Design review of the part built by this model. Coordinates are the model's own, in mm. Round coordinates to 2 decimals unless told otherwise and drop trailing zeros. Order: outer loops, then holes, each group sorted by start corner. A loop starts at its lowest first (then second) coordinate and runs counter-clockwise, first axis right, second up. Notation, with made-up numbers: M 37,5.25 L 41,5.25 A29 cw 41,33.25 Z; hole C 55,1.25 d9. An arc over 180 degrees is marked long. Write each question's results on one line, items separated by ' | '. Start each with the question number.
Item 1: Take a section at A-A, the plane x = 20.5. Write out the cut boundary in (y, z), plus the area to 3 significant figures.
Item 2: Take a section at B-B, the plane y = -41. Write out the cut boundary in (x, z) (3 decimals).
Item 3: Wall thickness on line 1 (X direction, y = 40, z = 2.5); line 2 (Y direction, x = 41.5, z = 4.5): over which ranges is each line inside the solid? List them lowest first. Write a range as [from, to].
Item 4: Clearance check with flat-ended pins moving along their axes: pin 1 (10 mm diameter, centred on x = -17, y = 2, fed in from -Z); pin 2 (3 mm diameter, centred on x = 41, y = 41, fed in from +Z). State where each tip first meets the part, or that it passes through.
```python
from build123d import *

# Parameters (mm, degrees)
F0_R     = 1.725
F0_W     = 3.5
F0_H     = 3.5
F1_DEPTH = 10


with BuildPart() as f1:
    # F0 (on Top) → F1 (new body)
    with BuildSketch(Plane.XY):
        Polygon((45, -45), (45, 0), (45, 45), (0, 45), (-45, 45), (-45, 0), (-45, -45), (0, -45), align=None)
        with Locations((-41, -41)):
            Circle(F0_R, mode=Mode.SUBTRACT)
        with Locations((-20, -20)):
            Rectangle(F0_W, F0_H, mode=Mode.SUBTRACT)
        with Locations((41, -41)):
            Circle(F0_R, mode=Mode.SUBTRACT)
        with Locations((20, -20)):
            Rectangle(F0_W, F0_H, mode=Mode.SUBTRACT)
        with Locations((-20, 20)):
            Rectangle(F0_W, F0_H, mode=Mode.SUBTRACT)
        with Locations((-41, 41)):
            Circle(F0_R, mode=Mode.SUBTRACT)
        with Locations((20, 20)):
            Rectangle(F0_W, F0_H, mode=Mode.SUBTRACT)
        with Locations((41, 41)):
            Circle(F0_R, mode=Mode.SUBTRACT)
    extrude(amount=F1_DEPTH)


solid = f1.part
```
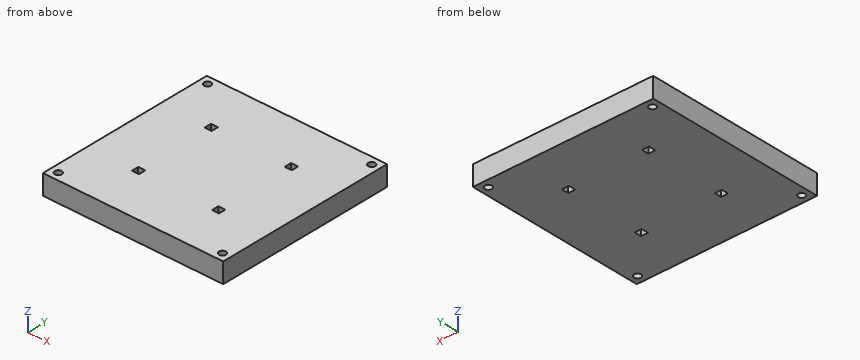
Results list:
1) outline: M -45,0 L -21.75,0 L -21.75,10 L -45,10 Z; M -18.25,0 L 18.25,0 L 18.25,10 L -18.25,10 Z; M 21.75,0 L 45,0 L 45,10 L 21.75,10 Z | area: 830 mm²
2) outline: M -45,0 L -42.725,0 L -42.725,10 L -45,10 Z; M -39.275,0 L 39.275,0 L 39.275,10 L -39.275,10 Z; M 42.725,0 L 45,0 L 45,10 L 42.725,10 Z
3) line 1: [-45, -42.41], [-39.59, 39.59], [42.41, 45] | line 2: [-45, -42.65], [-39.35, 39.35], [42.65, 45]
4) pin 1: z = 0 | pin 2: through
